Work out the finished part from the listing and answer in its coordinate system (mm). A direction names the side the tool comes from. Round coordinates to 2 decimals unless told otherwise and drop trailing zeros. Loops run counter-clockwise (first coordinate to the right, second up) from the corner with the lowest first, then second, coordinate; pieces in that order, holes last. Notation, with made-up numbers: (79, 4) -> (85, 4) arc R24 ccw to (85, 31) -> close; hole circle Ø11 at (36.5, -21). An arc over 180 degrees is marked (long way). Write item = value, one per line. Start each with the question number.
```python
from build123d import *

# Parameters (mm, degrees)
SKETCH_1_W               = 29
SKETCH_1_H               = 31.151212228
SKETCH_1_W_2             = 23
SKETCH_1_H_2             = 25.5
EXTRUDE_1_DEPTH          = 90
SKETCH_1_2_W             = 23
SKETCH_1_2_H             = 25.5
EXTRUDE_2_DEPTH          = 2
SKETCH_2_W               = 8
SKETCH_2_H               = 3
CUT_EXTRUDE_1_DEPTH      = 10
CUT_EXTRUDE_2_DEPTH      = 93.511147977
CUT_EXTRUDE_2_DEPTH_BACK = 93.511147977
FILLET_1_R               = 2
FILLET_2_R               = 1.5


with BuildPart() as part:
    # 스케치1 → 보스-돌출1 (new body)
    with BuildSketch(Plane.XY):
        with Locations((0, -0.174393886)):
            Rectangle(SKETCH_1_W, SKETCH_1_H)
        Rectangle(SKETCH_1_W_2, SKETCH_1_H_2, mode=Mode.SUBTRACT)
    extrude(amount=EXTRUDE_1_DEPTH)

    # 스케치1<2> → 보스-돌출2 (add)
    with BuildSketch(Plane.XY):
        Rectangle(SKETCH_1_2_W, SKETCH_1_2_H)
    extrude(amount=EXTRUDE_2_DEPTH)

    # 스케치2 → 컷-돌출1 (cut)
    with BuildSketch(Plane(origin=(0, 0, 0), x_dir=(-1, 0, 0), z_dir=(0, 0, -1))):
        with Locations((0, -14.25)):
            Rectangle(SKETCH_2_W, SKETCH_2_H)
    extrude(amount=-CUT_EXTRUDE_1_DEPTH, mode=Mode.SUBTRACT)

    # 스케치3 → 컷-돌출2 (cut, two sides: drawn at the far end of the back side and taken through both)
    with BuildSketch(Plane(origin=(0, 0, 0), x_dir=(1, 0, 0), z_dir=(0, 1, 0)).offset(-CUT_EXTRUDE_2_DEPTH_BACK)):
        Polygon((-9.5, -90), (-9.5, -86), (-11, -86), (-11, -83), (11, -83), (11, -86), (9.5, -86), (9.5, -90), align=None)
    extrude(amount=CUT_EXTRUDE_2_DEPTH + CUT_EXTRUDE_2_DEPTH_BACK, mode=Mode.SUBTRACT)

    # 필렛1
    fillet_1_edges = [part.edges().sort_by_distance(p)[0] for p in [
        (14.5, 15.401212228, 45),
        (14.5, -15.75, 45),
        (-14.5, -15.75, 45),
        (-14.5, 15.401212228, 45),
    ]]
    fillet(fillet_1_edges, radius=FILLET_1_R)

    # 필렛2
    fillet_2_edges = [part.edges().sort_by_distance(p)[0] for p in [
        (-11, -15.75, 90),
        (-8.25, -15.75, 0),
        (-14.5, -0.174393886, 0),
        (0, 15.401212228, 0),
        (14.5, -0.174393886, 0),
        (-13.914213562, 14.81542579, 0),
        (13.914213562, 14.81542579, 0),
        (13.914213562, -15.164213562, 0),
        (-13.914213562, -15.164213562, 0),
        (-14.5, -0.174393886, 90),
        (-13.914213562, 14.81542579, 90),
        (-13.914213562, -15.164213562, 90),
        (14.5, -0.174393886, 90),
        (11, 15.401212228, 90),
        (13.914213562, 14.81542579, 90),
        (13.914213562, -15.164213562, 90),
        (8.25, -15.75, 0),
        (11, -15.75, 90),
        (-11, 15.401212228, 90),
    ]]
    fillet(fillet_2_edges, radius=FILLET_2_R)


solid = part.part
```
Item 1: The mould has two halves that part along X. Classify faces 5 (the flat face through (-14.5, 0, 44)), 6 (the flat face through (11, -14, 84)), 7 (the cylindrical face through (-10.98, -15.32, 89.55)), 8 (the flat face through (14.5, 0, 44)): pulls with the +X half, pulls with the -X half, needs draft (parallel to the pull), parting line crosses it, or undercut.
Item 2: Section C-C (y = 5) is taken. Determine the outline of the cut face in (x, z), then the cut area to 3 significant figures.
Item 3: Find the intervals of material crossed by line 1 along X through (y, z) = (12, 60.5); line 2 along Y through (x, z) = (-8.25, 11.5); line 3 along Z through (x, y) = (3, 11), in increasing order. Write a range as [from, to].
Item 4: Flat-ended cylindrical pins translate along their axes: pin 1 (0.9 mm diameter, centred on y = -14.5, z = 4.5, fed in from +X); pin 2 (4 mm diameter, centred on x = 2.5, y = -8.5, fed in from +Z); pin 3 (1.6 mm diameter, centred on x = -1.5, z = 1.5, fed in from -Y). Find the tip coordinate at first contact, or state that the pin passes through.
Item 5: Section D-D (x = -5.5) is taken. Determine the outline of the cut face in (y, z), then the cut area to 3 significant figures.
Item 6: A tool of negligible diameter and unlimited length cuts with its end or side. For faces 1 (the flat face through (0, -14, 10)), 2 (the flat face through (0, 12.75, 36)), 3 (the flat face through (9.5, -14, 88)), 4 (the flat face through (-11, -14, 85)), from which of +Z, -Z, +X, -X, +Y, -Y can it reach the whole face along a straight path? Write none if from no direction.
Item 7: Section B-B (z = 58) is taken. Determine the outline of the cut face in (x, y), then the cut area to 3 significant figures.
Item 8: Section A-A (x = -0.75) is taken. Determine the outline of the cut face in (y, z).
Worked answers:
q1.face_5 = pulls with the -X half
q1.face_6 = undercut
q1.face_7 = needs draft
q1.face_8 = pulls with the +X half
q2.outline = (-14.5, 1.5) arc R1.5 ccw to (-13, 0) -> (13, 0) arc R1.5 ccw to (14.5, 1.5) -> (14.5, 88.5) arc R1.5 ccw to (13, 90) -> (11.5, 90) -> (11.5, 2) -> (-11.5, 2) -> (-11.5, 90) -> (-13, 90) arc R1.5 ccw to (-14.5, 88.5) -> close
q2.area = 584 mm2
q3.line_1 = [-14.5, -11.5], [11.5, 14.5]
q3.line_2 = [-15.75, -12.75], [12.75, 15.4]
q3.line_3 = [0, 2]
q4.pin_1 = 14.48
q4.pin_2 = 2
q4.pin_3 = -12.75
q5.outline = (-15.75, 1.5) arc R1.5 ccw to (-14.25, 0) -> (13.9, 0) arc R1.5 ccw to (15.4, 1.5) -> (15.4, 83) -> (12.75, 83) -> (12.75, 2) -> (-12.75, 2) -> (-12.75, 83) -> (-15.75, 83) -> close
q5.area = 519 mm2
q6.face_1 = -Z, -Y
q6.face_2 = +Z
q6.face_3 = +Z, +Y, -Y
q6.face_4 = +Y, -Y
q7.outline = (-14.5, -13.75) arc R2 ccw to (-12.5, -15.75) -> (12.5, -15.75) arc R2 ccw to (14.5, -13.75) -> (14.5, 13.4) arc R2 ccw to (12.5, 15.4) -> (-12.5, 15.4) arc R2 ccw to (-14.5, 13.4) -> close; hole (-11.5, -12.75) -> (11.5, -12.75) -> (11.5, 12.75) -> (-11.5, 12.75) -> close
q7.area = 313 mm2
q8.outline = (-15.75, 10) -> (-12.75, 10) -> (-12.75, 83) -> (-15.75, 83) -> close; (-12.75, 0) -> (13.9, 0) arc R1.5 ccw to (15.4, 1.5) -> (15.4, 83) -> (12.75, 83) -> (12.75, 2) -> (-12.75, 2) -> close
